The listing builds one solid part. Answer for the finished solid, in the listing's coordinates (mm). Face numbers are marked on the shaded views. A direction names the side the tool comes from. Coordinates: 2 decimals unless noted, no trailing zeros. Order: outer loops, then holes, each group sorted by start corner. A loop starts at its lowest first (then second) coordinate and runs counter-clockwise, first axis right, second up. Notation, with made-up numbers: (-32.5, -17) -> (-24.5, -17) arc R14 cw to (-24.5, 3) -> close; hole circle Ø7 at (21.5, 73). An arc over 180 degrees is marked (long way). Answer in a Markdown table with one row per item.
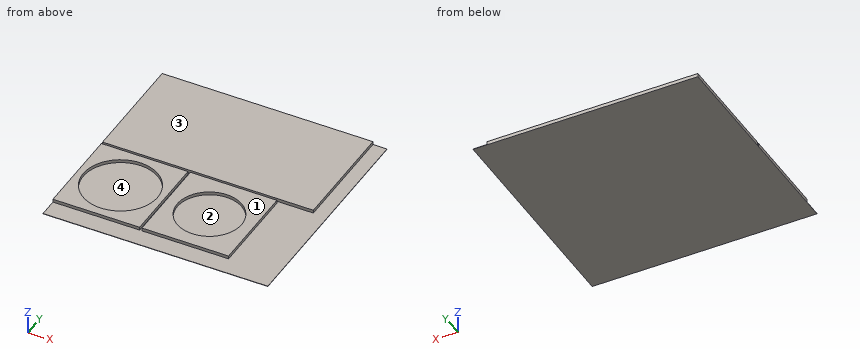
```python
from build123d import *

# Parameters (mm, degrees)
F0_W     = 1219.2
F0_H     = 1219.2
F1_DEPTH = 19.05
F2_W     = 469.9
F2_H     = 495.3
F3_DEPTH = 17.145
F4_R     = 201.6125
F5_DEPTH = 17.145
F6_R     = 174.625
F7_DEPTH = 17.145


with BuildPart() as f1:
    # F0 (on Top) → F1 (new body)
    with BuildSketch(Plane.XY):
        Rectangle(F0_W, F0_H)
    extrude(amount=F1_DEPTH)

    # F2 (on face) → F3 (cut)
    with BuildSketch(Plane.XY.offset(19.05)):
        Polygon((609.6, 609.6), (533.4, 609.6), (533.4, 0), (-609.6, 0), (-609.6, -12.7), (-139.7, -12.7), (-139.7, -508), (-609.6, -508), (-609.6, -609.6), (609.6, -609.6), align=None)
        with Locations((107.95, -260.35)):
            Rectangle(F2_W, F2_H, mode=Mode.SUBTRACT)
    extrude(amount=-F3_DEPTH, mode=Mode.SUBTRACT)

    # F4 (on face) → F5 (cut)
    with BuildSketch(Plane.XY.offset(19.05)):
        with Locations((-374.65, -260.35)):
            Circle(F4_R)
    extrude(amount=-F5_DEPTH, mode=Mode.SUBTRACT)

    # F6 (on face) → F7 (cut)
    with BuildSketch(Plane.XY.offset(19.05)):
        with Locations((107.95, -260.35)):
            Circle(F6_R)
    extrude(amount=-F7_DEPTH, mode=Mode.SUBTRACT)


solid = f1.part
```
(1) A cutting plane is placed at A-A, the plane z = 15.5. Count the separate pieces of the cut face and the enclosed holes in it, then the cut area to 3 significant figures.
Check values:
| item | result |
|---|---|
| separate pieces | 3 |
| enclosed holes | 2 |
| area | 939,000 mm² |
(2) Flat-ended cylindrical pins translate along their axes: pin 1 (8.5 mm diameter, centred on y = -328.5, z = 10, fed in from +X); pin 2 (2 mm diameter, centred on x = 15.5, y = -253, fed in from -Z); pin 3 (5 mm diameter, centred on x = 165.5, z = 8.5, fed in from -Y). Find the tip coordinate at first contact, or state that the pin passes through.
Check values:
| item | result |
|---|---|
| pin 1 | x = 342.9 |
| pin 2 | z = 0 |
| pin 3 | y = -508 |
(3) Which of the six approach directions +Z, -Z, +X, -X, +Y, -Y give full straight-line access (tool end or side, diameter ignored) to the marked faces 1 and 2?
Check values:
| item | result |
|---|---|
| face 1 | +Z, +X, -X, +Y, -Y |
| face 2 | +Z |
(4) For a pull along Y with two mould halves and no side action, classify the marked faces 3 and 4 as released by +Y, released by -Y, zero draft, split by the parting line, or undercut.
Check values:
| item | result |
|---|---|
| face 3 | zero draft |
| face 4 | undercut |
(5) A cutting plane is placed at B-B, the plane x = 107.95. Determine the outline of the cut face in (y, z) (3 decimals), then the cut area to 3 significant figures.
Check values:
| item | result |
|---|---|
| outline | (-609.6, 0) -> (609.6, 0) -> (609.6, 19.05) -> (0, 19.05) -> (0, 1.905) -> (-12.7, 1.905) -> (-12.7, 19.05) -> (-85.725, 19.05) -> (-85.725, 1.905) -> (-434.975, 1.905) -> (-434.975, 19.05) -> (-508, 19.05) -> (-508, 1.905) -> (-609.6, 1.905) -> close |
| area | 15,300 mm² |
(6) Find the intervals of material crossed by line 1 along Y through (x, z) = (107.95, 11.5) (3 decimals); line 2 along Y through (x, z) = (-374.65, 7.25); line 3 along Y through (x, z) = (-125, 15.25), in increasing order. Write a range as from..to.
Check values:
| item | result |
|---|---|
| line 1 | -508..-434.975, -85.725..-12.7, 0..609.6 |
| line 2 | -508..-461.96, -58.74..-12.7, 0..609.6 |
| line 3 | -508..-12.7, 0..609.6 |
